Job drawing, mm, ordinate dimensions from the low corner. One solid piece. A direction names the side the tool comes from. Round coordinates to 2 decimals unless told otherwise and drop trailing zeros. Loops run counter-clockwise (first coordinate to the right, second up) from the corner with the lowest first, then second, coordinate; pieces in that order, holes last.
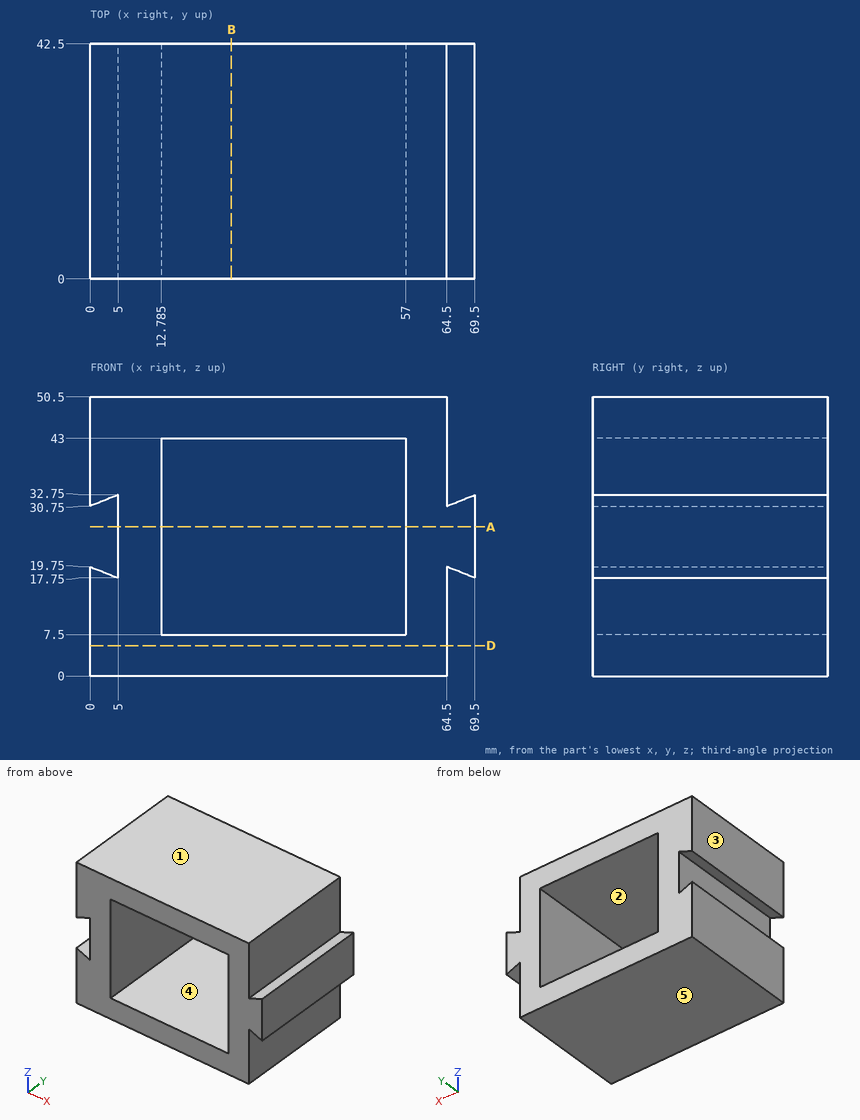
Item 1: 3-axis set-ups, long thin cutter, end or side, ignore diameter. For the marked faces 4 and 5: which of +Z, -Z, +X, -X, +Y, -Y reach the whole face in a straight line?
Answers follow:
face 4: +Y, -Y
face 5: -Z, +X, -X, +Y, -Y
Item 2: Cut at D-D, the plane z = 5.5. Give the cut face in (x, y).
Answers follow:
outline: (0, 0) - (64.5, 0) - (64.5, 42.5) - (0, 42.5) - close
Item 3: Cut at A-A, the plane z = 27. Give the cut face in (x, y) (1 decimal).
Answers follow:
outline: (5, 0) - (12.8, 0) - (12.8, 42.5) - (5, 42.5) - close; (57, 0) - (69.5, 0) - (69.5, 42.5) - (57, 42.5) - close
Item 4: Cut at B-B, the plane x = 25.5. Give the cut face in (y, z).
Answers follow:
outline: (0, 0) - (42.5, 0) - (42.5, 7.5) - (0, 7.5) - close; (0, 43) - (42.5, 43) - (42.5, 50.5) - (0, 50.5) - close
Item 5: Flat gauge pin, fed straight in: P1, Ø10, axis at y = 13.5, z = 6, coming from the +X side. Where does the tip first touch, or does it go through?
Answers follow:
P1: stops at x = 64.5
Item 6: Probe line 1 (X direction, y = 6, z = 13) (1 decimal); line 2 (Z direction, x = 38.5, y = 16); line 3 (X direction, y = 35.5, z = 23) (1 decimal). List the from-to ranges inside material, lowest first.
Answers follow:
line 1: x = 0 to 12.8, 57 to 64.5
line 2: z = 0 to 7.5, 43 to 50.5
line 3: x = 5 to 12.8, 57 to 69.5
Item 7: Two-plate mould, pull along Z, no slides. Class the marked faces 1, 2 and 3: released by +Z, released by -Z, zero draft, split by the parting line, or undercut.
Answers follow:
face 1: released by +Z
face 2: undercut
face 3: zero draft
